from build123d import *

# Parameters (mm, degrees)
STOCK_ACRYLIC_PARTS_1_OUTLINE_R   = 1.699983
STOCK_ACRYLIC_PARTS_1_OUTLINE_R_2 = 12
STOCK_ACRYLIC_PARTS_1_OUTLINE_R_3 = 2.1
STOCK_ACRYLIC_PARTS_1_OUTLINE_R_4 = 19
STOCK_ACRYLIC_PARTS_1_OUTLINE_R_5 = 1.55
STOCK_ACRYLIC_PARTS_1_OUTLINE_R_6 = 1.3
STOCK_ACRYLIC_PARTS_1_OUTLINE_R_7 = 1
STOCK_ACRYLIC_PARTS_1_OUTLINE_W   = 13
STOCK_ACRYLIC_PARTS_1_OUTLINE_H   = 7.6
STOCK_ACRYLIC_PARTS_1_OUTLINE_R_8 = 1.5
STOCK_ACRYLIC_PARTS_1_DEPTH       = 3
CUT_EXTRUDE1_DEPTH                = 10


# Read off the part's stored shape, not the designer's step: Stock-acrylic parts-1
with BuildPart() as part:
    # Stock-acrylic parts-1 outline → Stock-acrylic parts-1 (new body)
    with BuildSketch(Plane.XY):
        with BuildLine():
            ThreePointArc((821.147949544, 206.202079658), (824.798296467, 208.564256212), (824.138971465, 212.861953418))
            ThreePointArc((824.138971465, 212.861953418), (749.503192804, 246.381695406), (674.867414142, 212.861953418))
            ThreePointArc((674.867414142, 212.861953418), (674.208089141, 208.564256212), (677.858436064, 206.202079658))
            Line((677.858436064, 206.202079658), (681.094663275, 206.202079658))
            ThreePointArc((681.094663275, 206.202079658), (684.210031262, 204.911651986), (685.500458934, 201.796283999))
            Line((685.500458934, 201.796283999), (685.500458934, 140.108329038))
            ThreePointArc((685.500458934, 140.108329038), (684.209895956, 136.992634392), (681.09420131, 135.702071414))
            Line((681.09420131, 135.702071414), (677.866731501, 135.702071414))
            ThreePointArc((677.866731501, 135.702071414), (675.134308532, 134.625733906), (673.870013854, 131.975036511))
            Line((673.870013854, 131.975036511), (673.870013854, 118.558895729))
            ThreePointArc((673.870013854, 118.558895729), (693.951774589, 67.659471727), (744.285774281, 46.199812992))
            Line((744.285774281, 46.199812992), (749.503192804, 46.199785203))
            Line((749.503192804, 46.199785203), (754.720611326, 46.199812992))
            ThreePointArc((754.720611326, 46.199812992), (805.054611018, 67.659471727), (825.136371753, 118.558895729))
            Line((825.136371753, 118.558895729), (825.136371753, 131.975036511))
            ThreePointArc((825.136371753, 131.975036511), (823.872077075, 134.625733906), (821.139654106, 135.702071414))
            Line((821.139654106, 135.702071414), (817.912184297, 135.702071414))
            ThreePointArc((817.912184297, 135.702071414), (814.796489652, 136.992634392), (813.505926674, 140.108329038))
            Line((813.505926674, 140.108329038), (813.505926674, 201.796283999))
            ThreePointArc((813.505926674, 201.796283999), (814.796354345, 204.911651986), (817.911722332, 206.202079658))
            Line((817.911722332, 206.202079658), (821.147949544, 206.202079658))
        make_face()
        with Locations((734.502945377, 66.762651685)):
            Circle(STOCK_ACRYLIC_PARTS_1_OUTLINE_R, mode=Mode.SUBTRACT)
        with Locations((749.502795377, 66.762651685)):
            Circle(STOCK_ACRYLIC_PARTS_1_OUTLINE_R_2, mode=Mode.SUBTRACT)
        with BuildLine():
            Line((721.50260823, 73.962833599), (726.112087485, 73.962833599))
            ThreePointArc((726.112087485, 73.962833599), (726.502609759, 74.012836148), (726.893132033, 73.962833599))
            Line((726.893132033, 73.962833599), (731.502611288, 73.962833599))
            Line((731.502611288, 73.962833599), (731.502611288, 70.962833599))
            Line((731.502611288, 70.962833599), (726.893130503, 70.962838298))
            ThreePointArc((726.893130503, 70.962838298), (726.502608179, 70.912836148), (726.112085956, 70.962839094))
            Line((726.112085956, 70.962839094), (721.50260823, 70.962843794))
            Line((721.50260823, 70.962843794), (721.50260823, 73.962833599))
        make_face(mode=Mode.SUBTRACT)
        with Locations((689.120060972, 116.936022379)):
            Circle(STOCK_ACRYLIC_PARTS_1_OUTLINE_R_3, mode=Mode.SUBTRACT)
        with Locations((749.5, 129.5)):
            Circle(STOCK_ACRYLIC_PARTS_1_OUTLINE_R_4, mode=Mode.SUBTRACT)
        with Locations((764.502645377, 66.762651685)):
            Circle(STOCK_ACRYLIC_PARTS_1_OUTLINE_R, mode=Mode.SUBTRACT)
        with BuildLine():
            Line((767.502605171, 73.962833599), (772.112084426, 73.962833599))
            ThreePointArc((772.112084426, 73.962833599), (772.5026067, 74.012836148), (772.893128974, 73.962833599))
            Line((772.893128974, 73.962833599), (777.50260823, 73.962833599))
            Line((777.50260823, 73.962833599), (777.50260823, 70.962843794))
            Line((777.50260823, 70.962843794), (772.893130503, 70.962839094))
            ThreePointArc((772.893130503, 70.962839094), (772.50260828, 70.912836148), (772.112085956, 70.962838298))
            Line((772.112085956, 70.962838298), (767.502605171, 70.962833599))
            Line((767.502605171, 70.962833599), (767.502605171, 73.962833599))
        make_face(mode=Mode.SUBTRACT)
        with Locations((810.131525065, 116.936022379)):
            Circle(STOCK_ACRYLIC_PARTS_1_OUTLINE_R_3, mode=Mode.SUBTRACT)
        with Locations((694.236958178, 153.599764702)):
            Circle(STOCK_ACRYLIC_PARTS_1_OUTLINE_R_5, mode=Mode.SUBTRACT)
        with Locations((706.236958178, 153.599764702)):
            Circle(STOCK_ACRYLIC_PARTS_1_OUTLINE_R_5, mode=Mode.SUBTRACT)
        with Locations((694.236958178, 188.299764702)):
            Circle(STOCK_ACRYLIC_PARTS_1_OUTLINE_R_5, mode=Mode.SUBTRACT)
        with Locations((706.236958178, 188.299764702)):
            Circle(STOCK_ACRYLIC_PARTS_1_OUTLINE_R_5, mode=Mode.SUBTRACT)
        with BuildLine():
            Line((762.456929776, 167.185618031), (736.521624913, 167.180185031))
            ThreePointArc((736.521624913, 167.180185031), (733.487314362, 176.5518483), (736.51769824, 185.924782019))
            Line((736.51769824, 185.924782019), (762.453003098, 185.930215033))
            ThreePointArc((762.453003098, 185.930215033), (765.487313655, 176.558551758), (762.456929776, 167.185618031))
        make_face(mode=Mode.SUBTRACT)
        with Locations((697.05410976, 216.862387)):
            Circle(STOCK_ACRYLIC_PARTS_1_OUTLINE_R_6, mode=Mode.SUBTRACT)
        with Locations((706.041717574, 219.927474111)):
            Circle(STOCK_ACRYLIC_PARTS_1_OUTLINE_R_6, mode=Mode.SUBTRACT)
        with Locations((725.070137431, 207.45155957)):
            Circle(STOCK_ACRYLIC_PARTS_1_OUTLINE_R_5, mode=Mode.SUBTRACT)
        with Locations((738.285350665, 200.947214569)):
            Circle(STOCK_ACRYLIC_PARTS_1_OUTLINE_R_5, mode=Mode.SUBTRACT)
        with Locations((729.080559, 222.300895)):
            Circle(STOCK_ACRYLIC_PARTS_1_OUTLINE_R_7, mode=Mode.SUBTRACT)
        with Locations((749.500559, 222.390895)):
            Rectangle(STOCK_ACRYLIC_PARTS_1_OUTLINE_W, STOCK_ACRYLIC_PARTS_1_OUTLINE_H, mode=Mode.SUBTRACT)
        with Locations((749.500364247, 239.307685207)):
            Circle(STOCK_ACRYLIC_PARTS_1_OUTLINE_R_8, mode=Mode.SUBTRACT)
        with Locations((792.763770316, 153.599764702)):
            Circle(STOCK_ACRYLIC_PARTS_1_OUTLINE_R_5, mode=Mode.SUBTRACT)
        with BuildLine():
            ThreePointArc((804.766598873, 155.149762121), (806.31942743, 153.599764702), (804.766598873, 152.049767283))
            ThreePointArc((804.766598873, 152.049767283), (803.213770316, 153.599764702), (804.766598873, 155.149762121))
        make_face(mode=Mode.SUBTRACT)
        with Locations((792.763770316, 188.299764702)):
            Circle(STOCK_ACRYLIC_PARTS_1_OUTLINE_R_5, mode=Mode.SUBTRACT)
        with BuildLine():
            ThreePointArc((804.766598873, 189.849762121), (806.31942743, 188.299764702), (804.766598873, 186.749767283))
            ThreePointArc((804.766598873, 186.749767283), (803.213770316, 188.299764702), (804.766598873, 189.849762121))
        make_face(mode=Mode.SUBTRACT)
        with Locations((760.685350665, 200.947214569)):
            Circle(STOCK_ACRYLIC_PARTS_1_OUTLINE_R_5, mode=Mode.SUBTRACT)
        with Locations((773.997959275, 207.45155957)):
            Circle(STOCK_ACRYLIC_PARTS_1_OUTLINE_R_5, mode=Mode.SUBTRACT)
        with Locations((769.890559, 222.300895)):
            Circle(STOCK_ACRYLIC_PARTS_1_OUTLINE_R_7, mode=Mode.SUBTRACT)
        with Locations((792.951231186, 219.927474111)):
            Circle(STOCK_ACRYLIC_PARTS_1_OUTLINE_R_6, mode=Mode.SUBTRACT)
        with Locations((801.938839, 216.862387)):
            Circle(STOCK_ACRYLIC_PARTS_1_OUTLINE_R_6, mode=Mode.SUBTRACT)
    extrude(amount=STOCK_ACRYLIC_PARTS_1_DEPTH)

    # Sketch1 → Cut-Extrude1 (cut)
    with BuildSketch(Plane.XY.offset(3)):
        with BuildLine():
            Line((714.154659638, 118.266857616), (724.054510642, 118.321172443))
            ThreePointArc((724.054510642, 118.321172443), (726.561350155, 115.841690031), (724.081867742, 113.334850517))
            Line((724.081867742, 113.334850517), (714.182016738, 113.28053569))
            ThreePointArc((714.182016738, 113.28053569), (711.675177225, 115.760018102), (714.154659638, 118.266857616))
        make_face()
    extrude(amount=-CUT_EXTRUDE1_DEPTH, mode=Mode.SUBTRACT)


solid = part.part
The listing builds one solid part. Answer for the finished solid, in the listing's coordinates (mm). A direction names the side the tool comes from. Round coordinates to 2 decimals unless told otherwise and drop trailing zeros. Order: outer loops, then holes, each group sorted by start corner. A loop starts at its lowest first (then second) coordinate and runs counter-clockwise, first axis right, second up. Notation, with made-up numbers: (12.5, 64.25) -> (67.5, 64.25) arc R17 ccw to (67.5, 95.25) -> close; hole circle Ø3 at (19.5, 22). An arc over 180 degrees is marked (long way). Write each question's results on one line, items separated by ' | '. Start each with the question number.
Q1. Find section A-A (y = 129.5). Determine the outline of the cut face in (x, z), then the cut area to 3 significant figures.
Q2. Which of the six approach directions +Z, -Z, +X, -X, +Y, -Y give full straight-line access (tool end or side, diameter ignored) to faces 4 (the cylindrical face through (684.244, 137.027, 1.479)), 5 (the cylindrical face through (814.762, 204.877, 1.479)), 6 (the cylindrical face through (808.465, 115.658, 1.479))?
Q3. Each of these flat-tipped pins is pushed along its axis until it touches: pin 1 (1.5 mm diameter, centred on x = 770.5, z = 2, fed in from -Y); pin 2 (4 mm diameter, centred on x = 810.13, y = 116.94, fed in from +Z); pin 3 (0.9 mm diameter, centred on y = 172, z = 1, fed in from -X); pin 4 (1.5 mm diameter, centred on x = 783.5, z = 2.5, fed in from +Y). Where does it stop, or does it pass through?
Q4. The mould has two halves that part along X. Classify faces 1 (the cylindrical face through (750.683, 246.375, 1.479)), 2 (the cylindrical face through (691.12, 117.57, 1.48)), 3 (the cylindrical face through (693.406, 68.226, 1.479)): pulls with the +X half, pulls with the -X half, needs draft (parallel to the pull), parting line crosses it, or undercut.
Q5. Find section B-B (y = 62.5). Determine the outline of the cut face in (x, z), then the cut area to 3 significant figures.
Q6. Straight lines are drawn through the part: probe 1 along X at (y, z) = (72, 1.45); probe 2 along Y at (x, z) = (725.5, 2.2); probe 3 along X at (y, z) = (114.5, 2). For each, find the intervals that lie inside material, in ascending order. Write a range as from..to.
Q7. Find section C-C (z = 1.7). Give the number of separate pieces and of enclosed holes in the cut face, then the cut area to 3 significant figures.
Worked answers:
1) outline: (673.87, 0) -> (730.5, 0) -> (730.5, 3) -> (673.87, 3) -> close; (768.5, 0) -> (825.14, 0) -> (825.14, 3) -> (768.5, 3) -> close | area: 340 mm2
2) face 4: +Z, -Z, -X | face 5: +Z, -Z, +X | face 6: +Z, -Z
3) pin 1: stops at y = 47.92 | pin 2: passes through | pin 3: stops at x = 685.5 | pin 4: stops at y = 240.68
4) face 1: parting line crosses it | face 2: undercut | face 3: pulls with the -X half
5) outline: (699.54, 0) -> (738.29, 0) -> (738.29, 3) -> (699.54, 3) -> close; (760.72, 0) -> (799.46, 0) -> (799.46, 3) -> (760.72, 3) -> close | area: 232 mm2
6) probe 1: x = 690.06..721.5, 731.5..738.71, 760.3..767.5, 777.5..808.94 | probe 2: y = 48.87..70.96, 73.96..113.79, 117.87..205.96, 208.94..243.45 | probe 3: x = 673.9..712.03, 726.18..737.84, 761.16..825.1
7) separate pieces: 1 | enclosed holes: 30 | area: 22,300 mm2
